The listing builds one solid part. Answer for the finished solid, in the listing's coordinates (mm). Face numbers are marked on the shaded views. A direction names the side the tool comes from. Round coordinates to 2 decimals unless told otherwise and drop trailing zeros. Loops run counter-clockwise (first coordinate to the right, second up) from the corner with the lowest first, then second, coordinate; pieces in that order, holes last. Notation, with made-up numbers: (-26, 29.5) -> (-18, 29.5) arc R36 cw to (-18, 64.5) -> close; hole circle Ø7 at (86.5, -28). An arc over 180 degrees is marked (long way). Write each question's results on one line, items separated by ' | '. Start each with the question number.
(1) The part is cut by section D-D (z = 26). Determine the outline of the cut face in (x, y), plus the area to 3 significant figures.
(2) Straight lines are drawn through the part: probe 1 along X at (y, z) = (2.9, 5); probe 2 along X at (y, z) = (1.65, 35); probe 3 along Y at (x, z) = (3, 33). For each, find the intervals that lie inside material, in ascending order.
(3) The part is cut by section C-C (y = 35). Determine the outline of the cut face in (x, z).
(4) The part is cut by section A-A (x = 14). Determine the outline of the cut face in (y, z).
(5) Flat-ended cylindrical pins translate along their axes: pin 1 (1 mm diameter, centred on x = 23, z = 21, fed in from -Y); pin 2 (6.5 mm diameter, centred on x = 14, z = 35, fed in from +Y); pin 3 (13 mm diameter, centred on y = 35, z = 20, fed in from +X). Find the tip coordinate at first contact, or state that the pin passes through.
(6) For the marked faces 1 and 2, determine the directions among +Z, -Z, +X, -X, +Y, -Y from which every point of the face is accessible in a straight line to the end or side of a thin tool.
(7) The part is cut by section B-B (z = 20). Determine the outline of the cut face in (x, y).
```python
from build123d import *

# Parameters (mm, degrees)
SKETCH1_W           = 50
SKETCH1_H           = 40
BOSS_EXTRUDE1_DEPTH = 5
SKETCH2_W           = 5
SKETCH2_H           = 40
BOSS_EXTRUDE2_DEPTH = 50
FILLET1_R           = 3
CUT_EXTRUDE1_REACH  = 86.41
SKETCH3_R           = 4
CUT_EXTRUDE2_REACH  = 86.41
SKETCH5_R           = 1.7
CUT_EXTRUDE3_REACH  = 83.24
SKETCH6_R           = 2


with BuildPart() as part:
    # Sketch1 → Boss-Extrude1 (new body)
    with BuildSketch(Plane(origin=(0, 0, 0), x_dir=(1, 0, 0), z_dir=(0, 1, 0))):
        with Locations((25, -20)):
            Rectangle(SKETCH1_W, SKETCH1_H)
    extrude(amount=BOSS_EXTRUDE1_DEPTH)

    # Sketch2 → Boss-Extrude2 (add)
    with BuildSketch(Plane(origin=(0, 5, 0), x_dir=(1, 0, 0), z_dir=(0, 1, 0))):
        with Locations((2.5, -20)):
            Rectangle(SKETCH2_W, SKETCH2_H)
    extrude(amount=BOSS_EXTRUDE2_DEPTH)

    # Fillet1
    fillet1_edges = [part.edges().sort_by_distance(p)[0] for p in [
        (5, 5, 20),
        (0, 0, 20),
    ]]
    fillet(fillet1_edges, radius=FILLET1_R)

    # Sketch3 → Cut-Extrude1 (cut, up to next)
    with BuildSketch(Plane.ZY, mode=Mode.PRIVATE) as cut_extrude1_sk1:
        with Locations((20, 35)):
            Circle(SKETCH3_R)
    cut_extrude1_tool1 = extrude(cut_extrude1_sk1.sketch, amount=-CUT_EXTRUDE1_REACH, mode=Mode.PRIVATE) & part.part
    add(cut_extrude1_tool1.solids().sort_by_distance((0, 35, 20))[0], mode=Mode.SUBTRACT)

    # Sketch5 → Cut-Extrude2 (cut, up to next)
    with BuildSketch(Plane.ZY, mode=Mode.PRIVATE) as cut_extrude2_sk1:
        with Locations((7, 35)):
            Circle(SKETCH5_R)
    cut_extrude2_tool1 = extrude(cut_extrude2_sk1.sketch, amount=-CUT_EXTRUDE2_REACH, mode=Mode.PRIVATE) & part.part
    # Sketch5 → Cut-Extrude2 (cut, up to next)
    with BuildSketch(Plane.ZY, mode=Mode.PRIVATE) as cut_extrude2_sk2:
        with Locations((33, 35)):
            Circle(SKETCH5_R)
    cut_extrude2_tool2 = extrude(cut_extrude2_sk2.sketch, amount=-CUT_EXTRUDE2_REACH, mode=Mode.PRIVATE) & part.part
    # Sketch5 → Cut-Extrude2 (cut, up to next)
    with BuildSketch(Plane.ZY, mode=Mode.PRIVATE) as cut_extrude2_sk3:
        with Locations((20, 48)):
            Circle(SKETCH5_R)
    cut_extrude2_tool3 = extrude(cut_extrude2_sk3.sketch, amount=-CUT_EXTRUDE2_REACH, mode=Mode.PRIVATE) & part.part
    # Sketch5 → Cut-Extrude2 (cut, up to next)
    with BuildSketch(Plane.ZY, mode=Mode.PRIVATE) as cut_extrude2_sk4:
        with Locations((20, 22)):
            Circle(SKETCH5_R)
    cut_extrude2_tool4 = extrude(cut_extrude2_sk4.sketch, amount=-CUT_EXTRUDE2_REACH, mode=Mode.PRIVATE) & part.part
    add(cut_extrude2_tool1.solids().sort_by_distance((0, 35, 7))[0], mode=Mode.SUBTRACT)
    add(cut_extrude2_tool2.solids().sort_by_distance((0, 35, 33))[0], mode=Mode.SUBTRACT)
    add(cut_extrude2_tool3.solids().sort_by_distance((0, 48, 20))[0], mode=Mode.SUBTRACT)
    add(cut_extrude2_tool4.solids().sort_by_distance((0, 22, 20))[0], mode=Mode.SUBTRACT)

    # Sketch6 → Cut-Extrude3 (cut, up to next)
    with BuildSketch(Plane(origin=(0, 5, 0), x_dir=(1, 0, 0), z_dir=(0, 1, 0)), mode=Mode.PRIVATE) as cut_extrude3_sk1:
        with Locations(Location((14, -5, 0), (0, 0, 270))):
            Circle(SKETCH6_R)
    cut_extrude3_tool1 = extrude(cut_extrude3_sk1.sketch, amount=-CUT_EXTRUDE3_REACH, mode=Mode.PRIVATE) & part.part
    # Sketch6 → Cut-Extrude3 (cut, up to next)
    with BuildSketch(Plane(origin=(0, 5, 0), x_dir=(1, 0, 0), z_dir=(0, 1, 0)), mode=Mode.PRIVATE) as cut_extrude3_sk2:
        with Locations(Location((14, -35, 0), (0, 0, 270))):
            Circle(SKETCH6_R)
    cut_extrude3_tool2 = extrude(cut_extrude3_sk2.sketch, amount=-CUT_EXTRUDE3_REACH, mode=Mode.PRIVATE) & part.part
    # Sketch6 → Cut-Extrude3 (cut, up to next)
    with BuildSketch(Plane(origin=(0, 5, 0), x_dir=(1, 0, 0), z_dir=(0, 1, 0)), mode=Mode.PRIVATE) as cut_extrude3_sk3:
        with Locations(Location((44, -5, 0), (0, 0, 270))):
            Circle(SKETCH6_R)
    cut_extrude3_tool3 = extrude(cut_extrude3_sk3.sketch, amount=-CUT_EXTRUDE3_REACH, mode=Mode.PRIVATE) & part.part
    # Sketch6 → Cut-Extrude3 (cut, up to next)
    with BuildSketch(Plane(origin=(0, 5, 0), x_dir=(1, 0, 0), z_dir=(0, 1, 0)), mode=Mode.PRIVATE) as cut_extrude3_sk4:
        with Locations(Location((44, -35, 0), (0, 0, 270))):
            Circle(SKETCH6_R)
    cut_extrude3_tool4 = extrude(cut_extrude3_sk4.sketch, amount=-CUT_EXTRUDE3_REACH, mode=Mode.PRIVATE) & part.part
    add(cut_extrude3_tool1.solids().sort_by_distance((14, 5, 5))[0], mode=Mode.SUBTRACT)
    add(cut_extrude3_tool2.solids().sort_by_distance((14, 5, 35))[0], mode=Mode.SUBTRACT)
    add(cut_extrude3_tool3.solids().sort_by_distance((44, 5, 5))[0], mode=Mode.SUBTRACT)
    add(cut_extrude3_tool4.solids().sort_by_distance((44, 5, 35))[0], mode=Mode.SUBTRACT)


solid = part.part
```
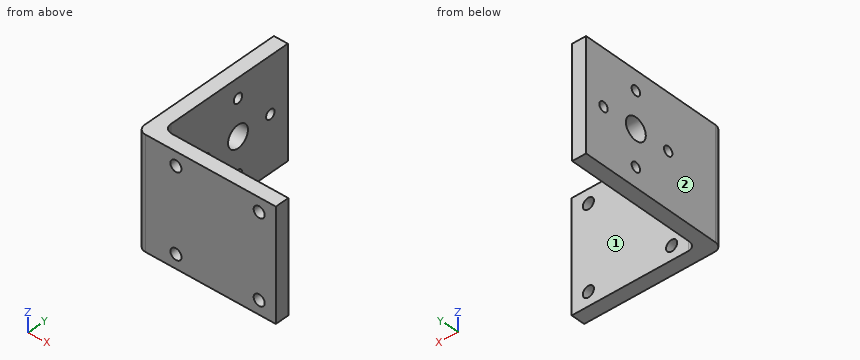
Checked values:
1) outline: (0, 3) arc R3 ccw to (3, 0) -> (50, 0) -> (50, 5) -> (8, 5) arc R3 cw to (5, 8) -> (5, 55) -> (0, 55) -> close | area: 500 mm2
2) probe 1: x = 0 to 12, 16 to 42, 46 to 50 | probe 2: x = 0.32 to 12, 16 to 42, 46 to 50 | probe 3: y = 0 to 33.3, 36.7 to 55
3) outline: (0, 0) -> (5, 0) -> (5, 5.3) -> (0, 5.3) -> close; (0, 8.7) -> (5, 8.7) -> (5, 16) -> (0, 16) -> close; (0, 24) -> (5, 24) -> (5, 31.3) -> (0, 31.3) -> close; (0, 34.7) -> (5, 34.7) -> (5, 40) -> (0, 40) -> close
4) outline: (0, 0) -> (5, 0) -> (5, 3) -> (0, 3) -> close; (0, 7) -> (5, 7) -> (5, 33) -> (0, 33) -> close; (0, 37) -> (5, 37) -> (5, 40) -> (0, 40) -> close
5) pin 1: stops at y = 0 | pin 2: stops at y = 5 | pin 3: stops at x = 5
6) face 1: +Z, -Z, +X, +Y | face 2: +Z, -Z, -X, +Y, -Y
7) outline: (0, 3) arc R3 ccw to (3, 0) -> (50, 0) -> (50, 5) -> (8, 5) arc R3 cw to (5, 8) -> (5, 20.3) -> (0, 20.3) -> close; (0, 23.7) -> (5, 23.7) -> (5, 31) -> (0, 31) -> close; (0, 39) -> (5, 39) -> (5, 46.3) -> (0, 46.3) -> close; (0, 49.7) -> (5, 49.7) -> (5, 55) -> (0, 55) -> close
